Read the model definition and answer for the solid it produces. Units are mm, in the model's axes. Face numbers are marked on the shaded views. A direction names the side the tool comes from. Coordinates: 2 decimals unless noted, no trailing zeros. Loops run counter-clockwise (first coordinate to the right, second up) from the corner with the lowest first, then second, coordinate; pieces in that order, holes last.
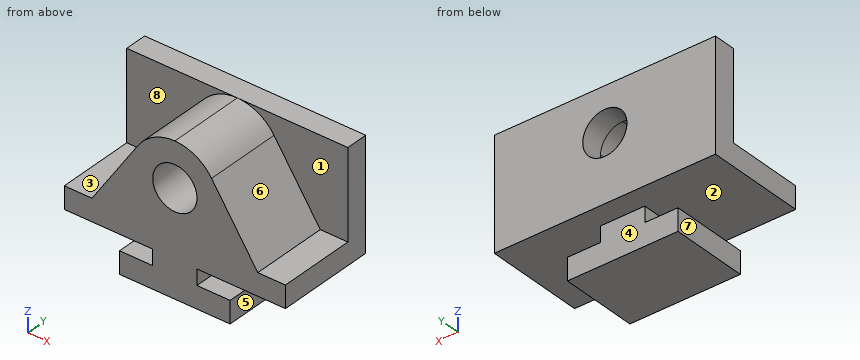
from build123d import *

# Parameters (mm, degrees)
F1_DEPTH = 44.45
F2_W     = 12.7
F2_H     = 63.5
F3_DEPTH = 158.75
F4_W     = 63.5
F4_H     = 63.5
F5_DEPTH = 50.8
F6_W     = 12.7
F6_H     = 63.5
F7_DEPTH = 31.75
F8_R     = 12.7
F9_DEPTH = 25.4


with BuildPart() as f1:
    # F0 (on Front) → F1 (new body)
    with BuildSketch(Plane.XZ):
        with BuildLine():
            ThreePointArc((44.45, 59.69), (40.730256, 68.670256), (31.75, 72.39))
            ThreePointArc((31.75, 72.39), (22.769744, 50.709744), (44.45, 59.69))
        make_face()
        with BuildLine():
            Line((0, 12.7), (0, 0))
            Line((0, 0), (63.5, 0))
            Line((63.5, 0), (63.5, 12.7))
            Line((63.5, 12.7), (44.45, 12.7))
            Line((44.45, 12.7), (44.45, 21.59))
            Line((44.45, 21.59), (95.25, 21.59))
            Line((95.25, 21.59), (95.25, 34.29))
            Line((95.25, 34.29), (79.375, 34.29))
            Line((79.375, 34.29), (52.843426, 73.840173))
            ThreePointArc((52.843426, 73.840173), (43.702941, 82.101765), (31.75, 85.09))
            ThreePointArc((31.75, 85.09), (19.797059, 82.101765), (10.656574, 73.840173))
            Line((10.656574, 73.840173), (-15.875, 34.29))
            Line((-15.875, 34.29), (-31.75, 34.29))
            Line((-31.75, 34.29), (-31.75, 21.59))
            Line((-31.75, 21.59), (19.05, 21.59))
            Line((19.05, 21.59), (19.05, 12.7))
            Line((19.05, 12.7), (0, 12.7))
        make_face()
        with BuildLine():
            ThreePointArc((44.45, 59.69), (22.769744, 50.709744), (31.75, 72.39))
            ThreePointArc((31.75, 72.39), (40.730256, 68.670256), (44.45, 59.69))
        make_face(mode=Mode.SUBTRACT)
    extrude(amount=F1_DEPTH)

    # F2 (on Right) → F3 (join)
    with BuildSketch(Plane.YZ):
        with Locations((6.35, 53.34)):
            Rectangle(F2_W, F2_H)
    extrude(amount=F3_DEPTH)

    # F4 (on face) → F5 (cut)
    with BuildSketch(Plane.XZ):
        with Locations((127, 53.34)):
            Rectangle(F4_W, F4_H)
    extrude(amount=-F5_DEPTH, mode=Mode.SUBTRACT)

    # F6 (on face) → F7 (join)
    with BuildSketch(Plane(origin=(0, 0, 0), x_dir=(0, -1, 0), z_dir=(-1, 0, 0))):
        with Locations((-6.35, 53.34)):
            Rectangle(F6_W, F6_H)
    extrude(amount=F7_DEPTH)

    # F8 (on face) → F9 (cut)
    with BuildSketch(Plane.XZ):
        with Locations((31.75, 59.69)):
            Circle(F8_R)
    extrude(amount=-F9_DEPTH, mode=Mode.SUBTRACT)


solid = f1.part
Q1. Determine the mould class of the marked faces 1, 2 and 3 for opening direction Z: +Z half, -Z half, draft (parallel to the pull), parting line (faces both ways), or undercut.
Findings below:
face 1: draft
face 2: undercut
face 3: +Z half
Q2. A cutting plane is placed at A-A (y = -28). Give the vertices of the cut face in (x, z) (3 decimals).
Findings below:
outline: (-31.75, 21.59) - (19.05, 21.59) - (19.05, 12.7) - (0, 12.7) - (0, 0) - (63.5, 0) - (63.5, 12.7) - (44.45, 12.7) - (44.45, 21.59) - (95.25, 21.59) - (95.25, 34.29) - (79.375, 34.29) - (52.843, 73.84) arc R25.4 ccw to (10.657, 73.84) - (-15.875, 34.29) - (-31.75, 34.29) - close; hole circle Ø25.4 at (31.75, 59.69)
Q3. A cutting plane is placed at B-B (z = 66.5). Give the vertices of the cut face in (x, y).
Findings below:
outline: (-31.75, 0) - (5.73, 0) - (5.73, -44.45) - (21.03, -44.45) - (21.03, 12.7) - (-31.75, 12.7) - close; (42.47, -44.45) - (57.77, -44.45) - (57.77, 0) - (95.25, 0) - (95.25, 12.7) - (42.47, 12.7) - close
Q4. A cutting plane is placed at C-C (x = 29). Give the vertices of the cut face in (y, z).
Findings below:
outline: (-44.45, 0) - (0, 0) - (0, 21.59) - (12.7, 21.59) - (12.7, 47.29) - (-44.45, 47.29) - close; (-44.45, 72.09) - (12.7, 72.09) - (12.7, 85.09) - (0, 85.09) - (0, 84.94) - (-44.45, 84.94) - close
Q5. Which of the six approach directions +Z, -Z, +X, -X, +Y, -Y give full straight-line access (tool end or side, diameter ignored) to the marked faces 4, 5, 6, 7 and 8?
Findings below:
face 4: -Z, +X, -X, +Y
face 5: -Z, +X, +Y, -Y
face 6: +Z, +X, -Y
face 7: -Z, -X, +Y, -Y
face 8: +Z, -X, -Y
Q6. Flat-ended cylindrical pins translate along their axes: pin 1 Ø6 at (x, y) = (70.5, -18) entering from +Z; pin 2 Ø20.5 at (x, z) = (31.75, 59.69) entering from +Y; pin 3 Ø3 at (y, z) = (-10.5, 36.5) entering from -X; pin 4 Ø15 at (x, y) = (49.5, -15) entering from +Z. Find the tip coordinate at first contact, or state that the pin passes through.
Findings below:
pin 1: stops at z = 51.99
pin 2: passes through
pin 3: stops at x = -15.4
pin 4: stops at z = 82.93
Q7. A cutting plane is placed at D-D (z = 45.5). Give the vertices of the cut face in (x, y), then the cut area to 3 significant figures.
Findings below:
outline: (-31.75, 0) - (-8.35, 0) - (-8.35, -44.45) - (71.85, -44.45) - (71.85, 0) - (95.25, 0) - (95.25, 12.7) - (-31.75, 12.7) - close
area: 5,180 mm2
Q8. Straight lines are drawn through the part: probe 1 along Z at (x, y) = (31.75, -28); probe 2 along Z at (x, y) = (31, 10); probe 3 along X at (y, z) = (9.25, 59.69). For each, find the intervals that lie inside material, in ascending order.
Findings below:
probe 1: z = 0 to 46.99, 72.39 to 85.09
probe 2: z = 21.59 to 47.01, 72.37 to 85.09
probe 3: x = -31.75 to 19.05, 44.45 to 95.25
